Part print with two shaded views. Sizes in mm from the minimum x, y, z corner. Round coordinates to 2 decimals unless told otherwise and drop trailing zeros. Loops run counter-clockwise (first coordinate to the right, second up) from the corner with the lowest first, then second, coordinate; pieces in that order, holes last.
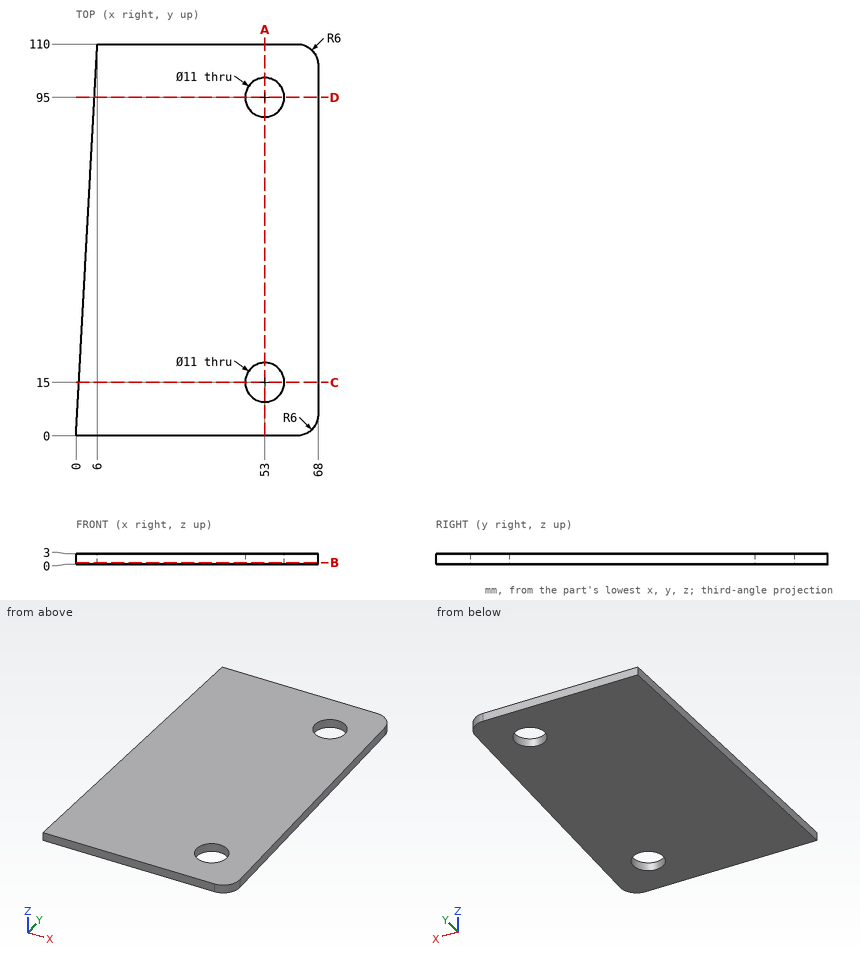
Item 1: Cut at A-A (x = 53). List the corners of the cut face in (y, z).
Verdict:
outline: (0, 0) - (9.5, 0) - (9.5, 3) - (0, 3) - close; (20.5, 0) - (89.5, 0) - (89.5, 3) - (20.5, 3) - close; (100.5, 0) - (110, 0) - (110, 3) - (100.5, 3) - close
Item 2: Flat gauge pins, fed straight in: P1, Ø1, axis at y = 70, z = 2, coming from the -X side; P2, Ø1, axis at y = 20, z = 1, coming from the -X side; P3, Ø1, axis at y = 83.5, z = 1, coming from the -X side. Where does each tip first touch, or does it go through?
Verdict:
P1: stops at x = 3.79
P2: stops at x = 1.06
P3: stops at x = 4.53
Item 3: Cut at B-B (z = 0.5). List the corners of the cut face in (x, y), plus the area to 3 significant figures.
Verdict:
outline: (0, 0) - (62, 0) arc R6 ccw to (68, 6) - (68, 104) arc R6 ccw to (62, 110) - (6, 110) - close; hole circle Ø11 at (53, 15); hole circle Ø11 at (53, 95)
area: 6,940 mm2
Item 4: Cut at C-C (y = 15). List the corners of the cut face in (x, z).
Verdict:
outline: (0.82, 0) - (47.5, 0) - (47.5, 3) - (0.82, 3) - close; (58.5, 0) - (68, 0) - (68, 3) - (58.5, 3) - close
Item 5: Wall check: L1, parallel to Y at x = 53, z = 1.45; L2, parallel to Y at x = 48, z = 0.25; L3, parallel to X at y = 18.5, z = 1. Give the ranges that are in metal, low to high.
Verdict:
L1: y = 0 to 9.5, 20.5 to 89.5, 100.5 to 110
L2: y = 0 to 12.71, 17.29 to 92.71, 97.29 to 110
L3: x = 1.01 to 48.76, 57.24 to 68
Item 6: Cut at D-D (y = 95). List the corners of the cut face in (x, z), plus the area to 3 significant figures.
Verdict:
outline: (5.18, 0) - (47.5, 0) - (47.5, 3) - (5.18, 3) - close; (58.5, 0) - (68, 0) - (68, 3) - (58.5, 3) - close
area: 155 mm2
